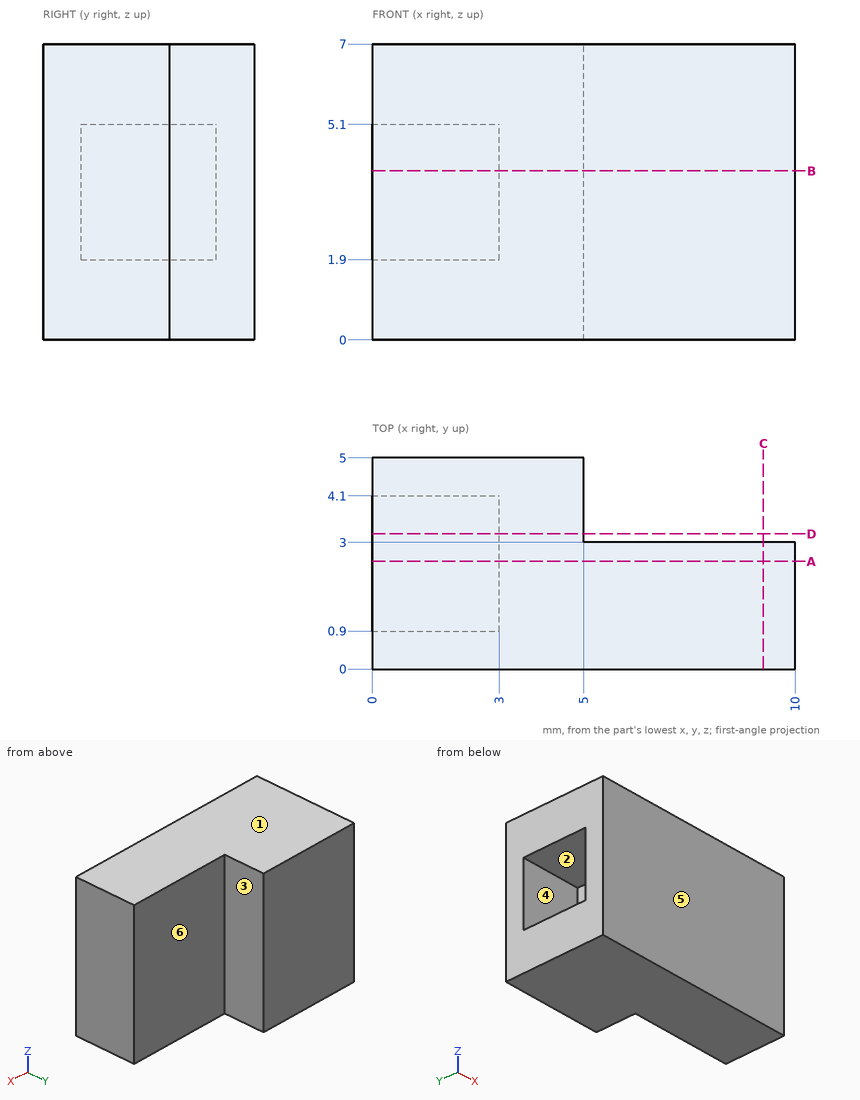
Design review of the part shown in the three views and the two pictorial views. Dimensions are in mm from the part's minimum x, y and z. A direction names the side the tool comes from. Coordinates: 2 decimals unless noted, no trailing zeros. Write each loop counter-clockwise with the first axis right and the second up, starting at its lowest first coordinate (ties: lowest second). Pieces come first, ordered by that corner, then holes.
(1) Wall thickness on probe 1 along Z at (x, y) = (0.5, 2.15); probe 2 along Y at (x, z) = (1.5, 2.25); probe 3 along Y at (x, z) = (7.75, 3): over which ranges is each line inside the solid? List them lowest first.
(2) Add section A-A on y = 2.55. Give the boundary of the cut face in (x, z), then the cut area to 3 significant figures.
(3) Tool access review of the marked faces 5 and 6: name each direction out of +Z, -Z, +X, -X, +Y, -Y from which nothing blocks a thin tool from reaching the whole face with its end or side.
(4) Add section C-C on x = 9.25. Give the boundary of the cut face in (y, z), then the cut area to 3 significant figures.
(5) For pin 1 Ø1.5 at (x, z) = (8, 4) entering from +Y; pin 2 Ø1 at (y, z) = (4, 4.5) entering from +X; pin 3 Ø1.6 at (y, z) = (3, 3.5) entering from -X, all flat-tipped, find the tip position at first contact; note any pin that passes through.
(6) Add section D-D on y = 3.2. Give the boundary of the cut face in (x, z), then the cut area to 3 significant figures.
(7) The part is to be moulded in two halves that separate along Z. For the marked faces 1, 2, 3 and 4, say which applies: +Z half, -Z half, draft (parallel to the pull), parting line (faces both ways), or undercut.
(8) Add section B-B on z = 4. Give the boundary of the cut face in (x, y), then the cut area to 3 significant figures.
Answer sheet:
1. probe 1: z = 0 to 1.9, 5.1 to 7
1. probe 2: y = 0 to 0.9, 4.1 to 5
1. probe 3: y = 0 to 3
2. outline: (0, 0) - (10, 0) - (10, 7) - (0, 7) - (0, 5.1) - (3, 5.1) - (3, 1.9) - (0, 1.9) - close
2. area: 60.4 mm2
3. face 5: +Z, -Z, +X, -X, -Y
3. face 6: +Z, -Z, +X, +Y
4. outline: (0, 0) - (3, 0) - (3, 7) - (0, 7) - close
4. area: 21.0 mm2
5. pin 1: stops at y = 3
5. pin 2: stops at x = 5
5. pin 3: stops at x = 3
6. outline: (0, 0) - (5, 0) - (5, 7) - (0, 7) - (0, 5.1) - (3, 5.1) - (3, 1.9) - (0, 1.9) - close
6. area: 25.4 mm2
7. face 1: +Z half
7. face 2: undercut
7. face 3: draft
7. face 4: undercut
8. outline: (0, 0) - (10, 0) - (10, 3) - (5, 3) - (5, 5) - (0, 5) - (0, 4.1) - (3, 4.1) - (3, 0.9) - (0, 0.9) - close
8. area: 30.4 mm2
